from build123d import *

# Parameters (mm, degrees)
F0_R     = 14.2875
F1_DEPTH = 39.624


with BuildPart() as f1:
    # F0 (on Front) → F1 (new body)
    with BuildSketch(Plane.XZ):
        with BuildLine():
            ThreePointArc((73.025, 0), (62.19921, 17.183273), (42.026063, 14.836624))
            ThreePointArc((42.026063, 14.836624), (34.934863, 0.612924), (41.096574, -14.037402))
            ThreePointArc((41.096574, -14.037402), (61.642088, -17.438987), (73.025, 0))
        make_face()
        with Locations((53.975, 0)):
            Circle(F0_R, mode=Mode.SUBTRACT)
        with BuildLine():
            ThreePointArc((14.607696, 24.559028), (24.838936, 14.126495), (28.575, 0))
            ThreePointArc((28.575, 0), (25.030648, -13.783951), (15.276852, -24.148466))
            Line((15.276852, -24.148466), (41.096574, -14.037402))
            ThreePointArc((41.096574, -14.037402), (34.934863, 0.612924), (42.026063, 14.836624))
            Line((42.026063, 14.836624), (14.607696, 24.559028))
        make_face()
        with BuildLine():
            ThreePointArc((15.276852, -24.148466), (25.030648, -13.783951), (28.575, 0))
            ThreePointArc((28.575, 0), (24.838936, 14.126495), (14.607696, 24.559028))
            ThreePointArc((14.607696, 24.559028), (-28.572304, -0.392534), (15.276852, -24.148466))
        make_face()
        with BuildLine():
            ThreePointArc((-13.470384, 4.7625), (0, 14.2875), (13.470384, 4.7625))
            Line((13.470384, 4.7625), (19.05, 4.7625))
            Line((19.05, 4.7625), (19.05, -4.7625))
            Line((19.05, -4.7625), (13.470384, -4.7625))
            ThreePointArc((13.470384, -4.7625), (0, -14.2875), (-13.470384, -4.7625))
            Line((-13.470384, -4.7625), (-19.05, -4.7625))
            Line((-19.05, -4.7625), (-19.05, 4.7625))
            Line((-19.05, 4.7625), (-13.470384, 4.7625))
        make_face(mode=Mode.SUBTRACT)
    extrude(amount=F1_DEPTH)


solid = f1.part
CAD build for the part. Positions are in the model's coordinates, mm. A direction names the side the tool comes from. Give positions to 0.01 mm unless a question says otherwise; leave off trailing zeros. Write each loop counter-clockwise with the first axis right and the second up, starting at its lowest first coordinate (ties: lowest second). Pieces come first, ordered by that corner, then holes. Notation, with made-up numbers: M -15.75,19 L 2.25,19 A28 ccw 2.25,53 Z; hole C 59.5,89.25 d6. An arc over 180 degrees is marked long. Put each result on its own line as item: value. Start each with the question number.
(1) Band-saw the part on D-D, the plane z = -12. Write the cut outline in (x, y), and give its area (3 significant figures).
(2) Which spindle directions (+Z, -Z, +X, -X, +Y, -Y) get a long thin tool onto all of the face, cutting with end or side? Do faces 5 (the face through (28.51, -19.53, 19.63)), 6 (the face through (0.246, -19.535, -14.285)), 7 (the face through (28.01, -19.53, -19.16)). Say none if no direction does.
(3) Band-saw the part on C-C, the plane z = 9. Write the cut outline in (x, y), and give its area (3 significant figures).
(4) Probe L1, parallel to X at y = -22, z = -1.5; L2, parallel to X at y = -5.5, z = 5; L3, parallel to Z at x = -10.5, y = -26. List the from-to ranges inside material, lowest first.
(5) Flat gauge pins, fed straight in: pin 1 Ø10 at (y, z) = (-23.5, -13.5) entering from -X; pin 2 Ø4.5 at (x, y) = (-15.5, -19.5) entering from +Z; pin 3 Ø6 at (x, y) = (15.5, -14) entering from -Z; pin 4 Ø17 at (x, z) = (53.975, 0) entering from -Y. Where does each tip first touch, or does it go through?
(6) Band-saw the part on A-A, the plane x = 0. Write the cut outline in (y, z) (1 decimal), and give its area (3 significant figures).
(7) Band-saw the part on B-B, the plane y = -5. Give the number of separate pieces and of enclosed holes in the cut face, and give its area (3 significant figures).
(8) Mould opens along Z. For faces 1 (the face through (-16, -20, -4.762)), 2 (the face through (16, -20, -4.762)), 3 (the face through (22, -39.624, 0)), 4 (the face through (-28.57, -19.53, 0.46)) say: +Z half, -Z half, draft (parallel to the pull), parting line (faces both ways), or undercut.
Response values:
1. outline: M -25.93,-39.62 L -7.75,-39.62 L -7.75,0 L -25.93,0 Z; M 7.75,-39.62 L 46.22,-39.62 L 46.22,0 L 7.75,0 Z; M 61.73,-39.62 L 68.77,-39.62 L 68.77,0 L 61.73,0 Z
1. area: 2,520 mm2
2. face 5: +Z, +Y, -Y
2. face 6: +Y, -Y
2. face 7: -Z, +Y, -Y
3. outline: M -27.12,-39.62 L -11.1,-39.62 L -11.1,0 L -27.12,0 Z; M 11.1,-39.62 L 42.88,-39.62 L 42.88,0 L 11.1,0 Z; M 65.07,-39.62 L 70.76,-39.62 L 70.76,0 L 65.07,0 Z
3. area: 2,120 mm2
4. L1: x = -28.54 to -19.05, 19.05 to 39.77, 68.18 to 72.97
4. L2: x = -28.13 to -13.38, 13.38 to 40.59, 67.36 to 72.36
4. L3: z = -26.58 to -9.69, 9.69 to 26.58
5. pin 1: stops at x = -27.28
5. pin 2: stops at z = 25.32
5. pin 3: stops at z = -25.7
5. pin 4: passes through
6. outline: M -39.6,-28.6 L 0,-28.6 L 0,-14.3 L -39.6,-14.3 Z; M -39.6,14.3 L 0,14.3 L 0,28.6 L -39.6,28.6 Z
6. area: 1,130 mm2
7. separate pieces: 1
7. enclosed holes: 2
7. area: 2,760 mm2
8. face 1: undercut
8. face 2: undercut
8. face 3: draft
8. face 4: parting line
